Can you work these out from the model? Positions are in its coordinate system, mm. A direction names the side the tool comes from. Give positions to 0.01 mm unless a question says otherwise; leave off trailing zeros. Loops run counter-clockwise (first coordinate to the right, second up) from the corner with the lowest first, then second, coordinate; pieces in that order, holes last. Notation, with made-up numbers: (24.5, 30) - (60.5, 30) arc R13 cw to (60.5, 45) - close; hole circle Ø2 at (19.25, 86.25). An arc over 180 degrees is marked (long way). Use a Markdown table: item, result. Add a question column.
```python
from build123d import *

# Parameters (mm, degrees)
ESBO_O1_W                = 200
ESBO_O1_H                = 180
RESSALTO_EXTRUS_O1_DEPTH = 26.5
CHANFRO1_SIZE            = 30
CASCA1_T                 = -2
ESBO_O2_W                = 105
ESBO_O2_H                = 53
CORTE_EXTRUS_O1_DEPTH    = 2
CAVIDADE1_START          = -100
CAVIDADE1_OUTLINE_R      = 2.5
CAVIDADE1_DEPTH          = 200


# Read off the part's stored shape, not the designer's step: Cavidade1
with BuildPart() as part:
    # Esboço1 → Ressalto-extrusão1 (new, symmetric)
    with BuildSketch(Plane(origin=(0, 0, 0), x_dir=(1, 0, 0), z_dir=(0, 1, 0))):
        Rectangle(ESBO_O1_W, ESBO_O1_H)
    extrude(amount=RESSALTO_EXTRUS_O1_DEPTH, both=True)

    # Chanfro1
    chanfro1_edges = [part.edges().sort_by_distance(p)[0] for p in [
        (100, 0, 90),
        (-100, 0, 90),
        (-100, 0, -90),
        (100, 0, -90),
    ]]
    chamfer(chanfro1_edges, length=CHANFRO1_SIZE)

    # Casca1
    casca1_openings = [part.faces().sort_by_distance(p)[0] for p in [
        (0, 26.5, 0),
        (0, -26.5, 0),
    ]]
    offset(amount=CASCA1_T, openings=casca1_openings, kind=Kind.INTERSECTION)

    # Esboço2 → Corte-extrusão1 (cut)
    with BuildSketch(Plane.XY.offset(90)):
        Rectangle(ESBO_O2_W, ESBO_O2_H)
    extrude(amount=-CORTE_EXTRUS_O1_DEPTH, mode=Mode.SUBTRACT)

    # Cavidade1 outline → Cavidade1 (cut)
    with BuildSketch(Plane.YZ.offset(CAVIDADE1_START)):
        with Locations((-1.25, 12)):
            Circle(CAVIDADE1_OUTLINE_R)
    extrude(amount=CAVIDADE1_DEPTH, mode=Mode.SUBTRACT)


solid = part.part
```
1. Will these pins go through, and if not, where does the flat tip stop? P1, Ø4.5, axis at y = -1.25, z = 12, coming from the -X side; P2, Ø2, axis at y = 4, z = 89.5, coming from the +X side; P3, Ø0.6, axis at y = -1, z = 89.5, coming from the -X side; P4, Ø6.5, axis at y = -1.25, z = 12, coming from the -X side.
2. On a 3-axis mill with a long thin cutter (end or side, diameter ignored), from which of +Z, -Z, +X, -X, +Y, -Y can I reach the whole of each face in a straight line? I mean faces 1 (the face through (85, 0, 75)), 2 (the face through (61, 0, 88)). Say none if no direction works.
3. Suppose I cut it at A-A (y = -1.25). List the corners of the cut face in (x, z) for me, and give its area (3 significant figures).
4. If we mould it in two halves opening along X, with no side actions, what happens to faces 3 (the face through (-85, 0, 75)), 4 (the face through (-83.38, 0.37, -73.79)), 5 (the face through (85, 0, -75))? For each: released by +X, released by -X, zero draft, split by the parting line, or undercut.
5. Suppose I cut it at B-B (z = -4.5). List the corners of the cut face in (x, y) for me, and give its area (3 significant figures).
6. Please list where these lines run through material, in increasing order: line 1 along X through (y, z) = (12.5, 57); line 2 along Y through (x, z) = (-99, 12); line 3 along X through (y, z) = (11, -65). Write a range as [from, to].
7. Suppose I cut it at D-D (y = 11.5). List the corners of the cut face in (x, z) for me, and give its area (3 significant figures).
8. Suppose I cut it at C-C (x = 80). List the corners of the cut face in (y, z) for me.
Results below:
| question | item | result |
|---|---|---|
| 1 | P1 | through |
| 1 | P2 | x = 71.5 |
| 1 | P3 | x = -70.8 |
| 1 | P4 | x = -100 |
| 2 | face 1 | +Z, +X, +Y, -Y |
| 2 | face 2 | +Y, -Y |
| 3 | outline | (-100, -60) - (-70, -90) - (70, -90) - (100, -60) - (100, 9.5) - (98, 9.5) - (98, -59.17) - (69.17, -88) - (-69.17, -88) - (-98, -59.17) - (-98, 9.5) - (-100, 9.5) - close; (-100, 14.5) - (-98, 14.5) - (-98, 59.17) - (-69.17, 88) - (-52.5, 88) - (-52.5, 90) - (-70, 90) - (-100, 60) - close; (52.5, 88) - (69.17, 88) - (98, 59.17) - (98, 14.5) - (100, 14.5) - (100, 60) - (70, 90) - (52.5, 90) - close |
| 3 | area | 1,140 mm² |
| 4 | face 3 | released by -X |
| 4 | face 4 | undercut |
| 4 | face 5 | released by +X |
| 5 | outline | (-100, -26.5) - (-98, -26.5) - (-98, 26.5) - (-100, 26.5) - close; (98, -26.5) - (100, -26.5) - (100, 26.5) - (98, 26.5) - close |
| 5 | area | 212 mm² |
| 6 | line 1 | [-100, -98], [98, 100] |
| 6 | line 2 | [-26.5, -3.75], [1.25, 26.5] |
| 6 | line 3 | [-95, -92.17], [92.17, 95] |
| 7 | outline | (-100, -60) - (-70, -90) - (70, -90) - (100, -60) - (100, 60) - (70, 90) - (52.5, 90) - (52.5, 88) - (69.17, 88) - (98, 59.17) - (98, -59.17) - (69.17, -88) - (-69.17, -88) - (-98, -59.17) - (-98, 59.17) - (-69.17, 88) - (-52.5, 88) - (-52.5, 90) - (-70, 90) - (-100, 60) - close |
| 7 | area | 1,160 mm² |
| 8 | outline | (-26.5, -80) - (26.5, -80) - (26.5, -77.17) - (-26.5, -77.17) - close; (-26.5, 77.17) - (26.5, 77.17) - (26.5, 80) - (-26.5, 80) - close |
